```python
from build123d import *

# Parameters (mm, degrees)
SKETCH1_W           = 25
SKETCH1_H           = 25
SKETCH1_W_2         = 23
SKETCH1_H_2         = 23
BOSS_EXTRUDE1_DEPTH = 200
SKETCH3_R           = 2
CUT_EXTRUDE1_DEPTH  = 25


with BuildPart() as part:
    # Sketch1 → Boss-Extrude1 (new body)
    with BuildSketch(Plane(origin=(0, 0, 0), x_dir=(1, 0, 0), z_dir=(0, 1, 0))):
        Rectangle(SKETCH1_W, SKETCH1_H)
        Rectangle(SKETCH1_W_2, SKETCH1_H_2, mode=Mode.SUBTRACT)
    extrude(amount=BOSS_EXTRUDE1_DEPTH)

    # Sketch2 → Revolve1 (revolve)
    with BuildSketch(Plane(origin=(0, -10, 0), x_dir=(-1, 0, 0), z_dir=(0, -1, 0))):
        with BuildLine():
            Line((0, 19), (0, 20))
            ThreePointArc((0, 20), (-20, 0), (0, -20))
            Line((0, -20), (0, -19))
            ThreePointArc((0, -19), (-19, 0), (0, 19))
        make_face()
    revolve(axis=Axis((0, -10, -20), (0, 0, 1)))

    # Sketch3 → Cut-Extrude1 (cut)
    with BuildSketch(Plane(origin=(12.5, 0, 0), x_dir=(0, 0, -1), z_dir=(1, 0, 0))):
        with Locations((7.5, 190)):
            Circle(SKETCH3_R)
        with Locations((7.5, 180)):
            Circle(SKETCH3_R)
        with Locations((-7.5, 190)):
            Circle(SKETCH3_R)
        with Locations((-7.5, 180)):
            Circle(SKETCH3_R)
        with Locations((7.5, 170)):
            Circle(SKETCH3_R)
        with Locations((-7.5, 170)):
            Circle(SKETCH3_R)
    extrude(amount=-CUT_EXTRUDE1_DEPTH, mode=Mode.SUBTRACT)


solid = part.part
```
The listing builds one solid part. Answer for the finished solid, in the listing's coordinates (mm). A direction names the side the tool comes from. Round coordinates to 2 decimals unless told otherwise and drop trailing zeros. Write each loop counter-clockwise with the first axis right and the second up, starting at its lowest first coordinate (ties: lowest second). Pieces come first, ordered by that corner, then holes. Notation, with made-up numbers: (58, -20) -> (72, -20) arc R14 cw to (72, 0) -> close; hole circle Ø8 at (-11, -18). An arc over 180 degrees is marked (long way). Use CSV: the item, a comma, the result in double quotes. Start each with the question number.
(1) Section C-C on z = 1 is taken. Give the vertices of the cut face in (x, y).
(2) Section B-B on y = 170 is taken. Give the vertices of the cut face in (x, z).
(3) Each of these flat-tipped pins is pushed along its axis until it touches: pin 1 (1 mm diameter, centred on x = -3.5, z = -3.5, fed in from +Y); pin 2 (0.6 mm diameter, centred on x = -12.5, z = 12, fed in from -Y); pin 3 (10 mm diameter, centred on x = 8.5, y = 170.5, fed in from -Z); pin 4 (2.5 mm diameter, centred on y = 190, z = -7.5, fed in from -X). Where does it stop, or does it pass through?
(4) Consider L1, parallel to Z at x = 12, y = 170; L2, parallel to X at y = 58.5, z = -6. Determine where each line is inside the solid, lowest interval first. Write a range as from..to.
(5) Section A-A on y = 144 is taken. Give the vertices of the cut face in (x, z), then the cut area to 3 significant figures.
(6) The mould has two halves that part along Z. Classify faces 1 (the face through (-11.993, 168.226, -8.423)), 2 (the face through (0, 99, -12.5)), 3 (the face through (0, 99, 12.5)): released by +Z, released by -Z, zero draft, split by the parting line, or undercut.
(7) Which of the six approach directions +Z, -Z, +X, -X, +Y, -Y give full straight-line access (tool end or side, diameter ignored) to faces 4 (the face through (0, 2, 11.5)), 5 (the face through (11.5, 99, 0)), 6 (the face through (12.007, 188.226, -8.423))?
(8) Section D-D on z = -7.5 is taken. Count the separate pieces of the cut face and the enclosed holes in it, then the cut area to 3 significant figures.
A:
1,outline,"(-12.5, 5.58) arc R19.97 ccw (long way) to (12.5, 5.58) -> (12.5, 200) -> (11.5, 200) -> (11.5, 6.33) arc R19.97 ccw to (-11.5, 6.33) -> (-11.5, 200) -> (-12.5, 200) -> close; hole (-12.5, 0) -> (-12.5, 4.27) arc R18.97 ccw (long way) to (12.5, 4.27) -> (12.5, 0) -> (11.5, 0) -> (11.5, 5.09) arc R18.97 ccw to (-11.5, 5.09) -> (-11.5, 0) -> close"
2,outline,"(-12.5, -12.5) -> (12.5, -12.5) -> (12.5, -9.5) -> (11.5, -9.5) -> (11.5, -11.5) -> (-11.5, -11.5) -> (-11.5, -9.5) -> (-12.5, -9.5) -> close; (-12.5, -5.5) -> (-11.5, -5.5) -> (-11.5, 5.5) -> (-12.5, 5.5) -> close; (-12.5, 9.5) -> (-11.5, 9.5) -> (-11.5, 11.5) -> (11.5, 11.5) -> (11.5, 9.5) -> (12.5, 9.5) -> (12.5, 12.5) -> (-12.5, 12.5) -> close; (11.5, -5.5) -> (12.5, -5.5) -> (12.5, 5.5) -> (11.5, 5.5) -> close"
3,pin 1,"stops at y = 9.5"
3,pin 2,"stops at y = -20.49"
3,pin 3,"stops at z = -12.5"
3,pin 4,"passes through"
4,L1,"z = -12.5..-9.5, -5.5..5.5, 9.5..12.5"
4,L2,"x = -12.5..-11.5, 11.5..12.5"
5,outline,"(-12.5, -12.5) -> (12.5, -12.5) -> (12.5, 12.5) -> (-12.5, 12.5) -> close; hole (-11.5, -11.5) -> (11.5, -11.5) -> (11.5, 11.5) -> (-11.5, 11.5) -> close"
5,area,"96.0 mm²"
6,face 1,"undercut"
6,face 2,"released by -Z"
6,face 3,"released by +Z"
7,face 4,"none"
7,face 5,"+Y"
7,face 6,"+X, -X"
8,separate pieces,"7"
8,enclosed holes,"1"
8,area,"496 mm²"
